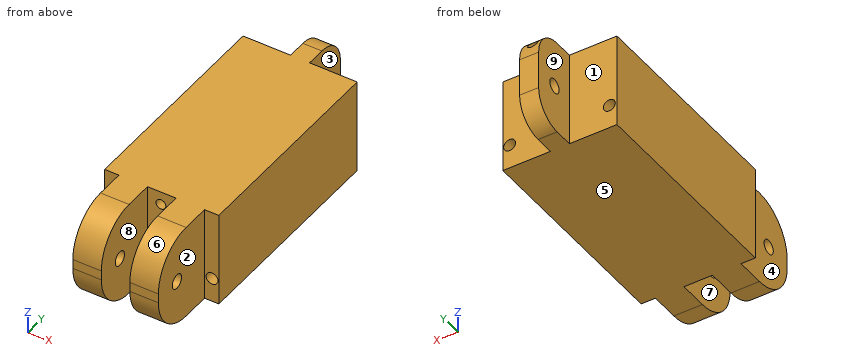
```python
from build123d import *

# Parameters (mm, degrees)
PAD_DEPTH       = 20
FILLET_R        = 9
FILLET001_R     = 9
FILLET002_R     = 9
FILLET003_R     = 9
FILLET004_R     = 6
FILLET005_R     = 6
SKETCH002_R     = 1.5
POCKET001_DEPTH = 14.001
SKETCH003_R     = 1.5
POCKET_DEPTH    = 21.001
SKETCH004_R     = 1.25
POCKET002_DEPTH = 55.001
SKETCH005_R     = 1.031889
POCKET003_DEPTH = 55.001


with BuildPart() as part:
    # Sketch → Pad (new body)
    with BuildSketch(Plane.XY):
        Polygon((-56.419573, 26.722219), (-46.419573, 26.722219), (-46.419573, 36.722219), (-42.419573, 36.722219), (-42.419573, 26.722219), (-32.419573, 26.722219), (-32.419573, -18.277781), (-35.419573, -18.277781), (-35.419573, -33.277781), (-41.419573, -33.277781), (-41.419573, -18.277781), (-47.419573, -18.277781), (-47.419573, -33.277781), (-53.419573, -33.277781), (-53.419573, -18.277781), (-56.419573, -18.277781), align=None)
    extrude(amount=PAD_DEPTH)

    # Fillet
    fillet_edges = [part.edges().sort_by_distance(p)[0] for p in [
        (-50.419573, -33.277781, 0),
    ]]
    fillet(fillet_edges, radius=FILLET_R)

    # Fillet001
    fillet001_edges = [part.edges().sort_by_distance(p)[0] for p in [
        (-50.419573, -33.277781, 20),
    ]]
    fillet(fillet001_edges, radius=FILLET001_R)

    # Fillet002
    fillet002_edges = [part.edges().sort_by_distance(p)[0] for p in [
        (-38.419573, -33.277781, 20),
    ]]
    fillet(fillet002_edges, radius=FILLET002_R)

    # Fillet003
    fillet003_edges = [part.edges().sort_by_distance(p)[0] for p in [
        (-38.419573, -33.277781, 0),
    ]]
    fillet(fillet003_edges, radius=FILLET003_R)

    # Fillet004
    fillet004_edges = [part.edges().sort_by_distance(p)[0] for p in [
        (-44.419573, 36.722219, 20),
    ]]
    fillet(fillet004_edges, radius=FILLET004_R)

    # Fillet005
    fillet005_edges = [part.edges().sort_by_distance(p)[0] for p in [
        (-44.419573, 36.722219, 0),
    ]]
    fillet(fillet005_edges, radius=FILLET005_R)

    # Sketch002 → Pocket001 (cut, through all)
    with BuildSketch(Plane.YZ.offset(-42.419573)):
        with Locations((31.587833, 9.786681)):
            Circle(SKETCH002_R)
    extrude(amount=-POCKET001_DEPTH, mode=Mode.SUBTRACT)

    # Sketch003 (on Face14 of Pocket001) → Pocket (cut, through all)
    with BuildSketch(Plane.YZ.offset(-35.419573)):
        with Locations((-27.264815, 9.786693)):
            Circle(SKETCH003_R)
    extrude(amount=-POCKET_DEPTH, mode=Mode.SUBTRACT)

    # Sketch004 (on Face15 of Pocket) → Pocket002 (cut, through all)
    with BuildSketch(Plane.XZ.offset(18.277781)):
        with Locations((-54.815166, 5.040761)):
            Circle(SKETCH004_R)
        with Locations((-33.842335, 5.136092)):
            Circle(SKETCH004_R)
    extrude(amount=-POCKET002_DEPTH, mode=Mode.SUBTRACT)

    # Sketch005 (on Face20 of Pocket002) → Pocket003 (cut, through all)
    with BuildSketch(Plane.XZ.offset(18.277781)):
        with Locations((-44.591709, 17.229778)):
            Circle(SKETCH005_R)
    extrude(amount=-POCKET003_DEPTH, mode=Mode.SUBTRACT)


solid = part.part
```
Work out the finished part from the listing and answer in its coordinate system (mm). Face numbers are marked on the shaded views. A direction names the side the tool comes from. Give positions to 0.01 mm unless a question says otherwise; leave off trailing zeros. Order: outer loops, then holes, each group sorted by start corner. A loop starts at its lowest first (then second) coordinate and runs counter-clockwise, first axis right, second up.
1. Section B-B, the plane y = 11 is taken. Determine the outline of the cut face in (x, z), and give its area (3 significant figures).
Result sheet:
outline: (-56.42, 0) - (-32.42, 0) - (-32.42, 20) - (-56.42, 20) - close; hole circle Ø2.5 at (-54.82, 5.04); hole circle Ø2.06 at (-44.59, 17.23); hole circle Ø2.5 at (-33.84, 5.14)
area: 467 mm2
2. The mould has two halves that part along X. Classify the marked faces 6, 7, 8 and 9: released by +X, released by -X, zero draft, split by the parting line, or undercut.
Result sheet:
face 6: zero draft
face 7: undercut
face 8: undercut
face 9: released by -X
3. Straight lines are drawn through the part: L1, parallel to Z at x = -33.75, y = -6.5; L2, parallel to X at y = 23, z = 5.5; L3, parallel to X at y = -7, z = 4.5. For each, find the intervals that lie inside material, in ascending order.
Result sheet:
L1: z = 0 to 3.89, 6.38 to 20
L2: x = -56.42 to -55.98, -53.65 to -35.04, -32.65 to -32.42
L3: x = -56.42 to -55.94, -53.69 to -34.92, -32.77 to -32.42
4. Section A-A, the plane x = -54.25 is taken. Determine the outline of the cut face in (y, z), and give its area (3 significant figures).
Result sheet:
outline: (-18.28, 0) - (26.72, 0) - (26.72, 3.93) - (-18.28, 3.93) - close; (-18.28, 6.16) - (26.72, 6.16) - (26.72, 20) - (-18.28, 20) - close
area: 800 mm2
5. For the marked faces 1, 2, 3, 4 and 5, determine the directions among +Z, -Z, +X, -X, +Y, -Y from which every point of the face is accessible in a straight line to the end or side of a thin tool.
Result sheet:
face 1: +Z, -Z, -X, +Y
face 2: +Z, -Z, +X, -Y
face 3: +Z, -Z, +X, +Y
face 4: +Z, -Z, -X, -Y
face 5: -Z, +X, -X, +Y, -Y
6. Section D-D, the plane z = 7 is taken. Determine the outline of the cut face in (x, y).
Result sheet:
outline: (-56.42, -18.28) - (-53.42, -18.28) - (-53.42, -33.05) - (-47.42, -33.05) - (-47.42, -18.28) - (-41.42, -18.28) - (-41.42, -33.05) - (-35.42, -33.05) - (-35.42, -18.28) - (-32.42, -18.28) - (-32.42, 26.72) - (-42.42, 26.72) - (-42.42, 36.72) - (-46.42, 36.72) - (-46.42, 26.72) - (-56.42, 26.72) - close
7. Section C-C, the plane x = -37.5 is taken. Determine the outline of the cut face in (y, z), and give its area (3 significant figures).
Result sheet:
outline: (-33.28, 9) arc R9 ccw to (-24.28, 0) - (26.72, 0) - (26.72, 20) - (-24.28, 20) arc R9 ccw to (-33.28, 11) - close; hole circle Ø3 at (-27.26, 9.79)
area: 1,160 mm2
8. Each of these flat-tipped pins is pushed along its axis until it touches: P1, Ø5, axis at y = -27.26, z = 9.79, coming from the -X side; P2, Ø3, axis at x = -53.5, z = 6.5, coming from the +Y side; P3, Ø8, axis at x = -47.5, z = 4, coming from the -Y side. Where does it stop, or does it pass through?
Result sheet:
P1: stops at x = -53.42
P2: stops at y = 26.72
P3: stops at y = -33.22
